Can you work these out from the model? Positions are in its coordinate system, mm. A direction names the side the tool comes from. Coordinates: 2 decimals unless noted, no trailing zeros. Order: outer loops, then holes, each group sorted by start corner. A loop starts at its lowest first (then second) coordinate and runs counter-clockwise, first axis right, second up. Notation, with made-up numbers: (86.25, 10) -> (118.25, 10) arc R10 ccw to (118.25, 25) -> close; hole circle Ø4 at (-5.75, 45). An arc over 180 degrees is marked (long way). Use a Markdown table: item, result. Add a question column.
1. Suppose I cut it at A-A, the plane x = 43.18. State how many separate pieces and enclosed holes the cut face has, then the cut area to 3 significant figures.
2. For faces 4 (the flat face through (-1, 10, 3.175)), 5 (the flat face through (-1, -10, 3.175)), 6 (the cylindrical face through (23.599, 0.022, 11.955)), which set-ups out of +Z, -Z, +X, -X, +Y, -Y let a thin tool reach every point of the face, with its end or its side?
3. If I drill on line 1 along X through (y, z) = (11, 1); line 2 along Y through (x, z) = (-43.18, 1.75) (3 decimals); line 3 along Y through (x, z) = (37.5, 14.5), over which ranges is the centre line in solid material (lowest first)? Write a range as from..to.
4. Suppose I cut it at D-D, the plane y = -3.5. List the corners of the cut face in (x, z) for me (3 decimals).
5. We'd pull the mould along Y, two halves only. Please class faces 1 (the flat face through (-1, 1.588, 35)), 2 (the flat face through (-1, 0, 66.675)), 3 (the cylindrical face through (-40.15, 12.38, 1.57)): pulls with the +Y half, pulls with the -Y half, needs draft (parallel to the pull), parting line crosses it, or undercut.
6. Suppose I cut it at B-B, the plane y = 11.43. List the corners of the cut face in (x, z) for me (3 decimals).
7. For pin 1 Ø2 at (y, z) = (-2.5, 28.5) entering from +X; pin 2 Ø5 at (x, y) = (43.18, 11.43) entering from -Z; pin 3 Ø6 at (x, z) = (-40, 55) entering from +Y; pin 4 Ø2 at (x, z) = (-31, 43.5) entering from -Y, each with a flat end and sliding along its axis, tell me the tip position at first contact or that it passes through.
```python
from build123d import *

# Parameters (mm, degrees)
F0_W     = 101.6
F0_H     = 38.1
F0_R     = 3.175
F1_DEPTH = 3.175
F2_W     = 101.6
F2_H     = 63.5
F2_R     = 1.37541
F3_DEPTH = 1.5875


with BuildPart() as f1:
    # F0 (on Top) → F1 (new body)
    with BuildSketch(Plane.XY):
        Rectangle(F0_W, F0_H)
        with Locations((-43.18, -11.43)):
            Circle(F0_R, mode=Mode.SUBTRACT)
        with Locations((43.18, -11.43)):
            Circle(F0_R, mode=Mode.SUBTRACT)
        with Locations((-43.18, 11.43)):
            Circle(F0_R, mode=Mode.SUBTRACT)
        with Locations((43.18, 11.43)):
            Circle(F0_R, mode=Mode.SUBTRACT)
    extrude(amount=F1_DEPTH)

    # F2 (on Front) → F3 (join, symmetric)
    with BuildSketch(Plane.XZ):
        with Locations((0, 34.925)):
            Rectangle(F2_W, F2_H)
        with Locations((-35.1409, 10.795)):
            Circle(F2_R, mode=Mode.SUBTRACT)
        with Locations((22.86, 10.795)):
            Circle(F2_R, mode=Mode.SUBTRACT)
        with Locations((-35.1409, 59.79414)):
            Circle(F2_R, mode=Mode.SUBTRACT)
        with Locations((22.86, 59.79414)):
            Circle(F2_R, mode=Mode.SUBTRACT)
    extrude(amount=F3_DEPTH, both=True)


solid = f1.part
```
Worked out:
| question | item | result |
|---|---|---|
| 1 | separate pieces | 3 |
| 1 | enclosed holes | 0 |
| 1 | area | 282 mm² |
| 2 | face 4 | +Z, +X, -X, +Y |
| 2 | face 5 | +Z, +X, -X, -Y |
| 2 | face 6 | +Y, -Y |
| 3 | line 1 | x = -50.8..-46.33, -40.03..40.03, 46.33..50.8 |
| 3 | line 2 | y = -19.05..-14.605, -8.255..8.255, 14.605..19.05 |
| 3 | line 3 | y = -1.59..1.59 |
| 4 | outline | (-50.8, 0) -> (50.8, 0) -> (50.8, 3.175) -> (-50.8, 3.175) -> close |
| 5 | face 1 | pulls with the +Y half |
| 5 | face 2 | needs draft |
| 5 | face 3 | undercut |
| 6 | outline | (-50.8, 0) -> (-46.355, 0) -> (-46.355, 3.175) -> (-50.8, 3.175) -> close; (-40.005, 0) -> (40.005, 0) -> (40.005, 3.175) -> (-40.005, 3.175) -> close; (46.355, 0) -> (50.8, 0) -> (50.8, 3.175) -> (46.355, 3.175) -> close |
| 7 | pin 1 | stops at x = 50.8 |
| 7 | pin 2 | passes through |
| 7 | pin 3 | stops at y = 1.59 |
| 7 | pin 4 | stops at y = -1.59 |
